Geometry: final body of the model. Coordinates: model frame, mm. A direction names the side the tool comes from. Coordinates: 2 decimals unless noted, no trailing zeros. Write each loop counter-clockwise with the first axis right and the second up, starting at its lowest first coordinate (ties: lowest second). Pieces come first, ordered by that corner, then holes. Notation, with made-up numbers: (64, -1) - (81, -1) arc R23 ccw to (81, 13) - close; hole circle Ø4 at (-30.5, 79.25). An arc over 180 degrees is marked (long way). Answer as a JSON object with one key per item and string values. Group by question number.
Item 1: Section C-C on x = -26.25. Return loops of the section in (y, z).
Item 2: Set-up query: faces 4 (the flat face through (0, 4, 2)), 5 (the cylindrical face through (-1.6, -25.9, 9.2)), 6 (the flat face through (-5, -15, 6)), 7 (the flat face through (-33, -15, 16)). Return all of +Z, -Z, +X, -X, +Y, -Y with unobstructed straight access to the full face (end or side cutting, diameter ignored); none if empty.
Item 3: Mould query, pull axis Z, two halves, no side actions, for faces 1 (the flat face through (-18, 5, 2)), 2 (the flat face through (-18, 4, 16)), 3 (the conical face through (-32.242, -21.255, 8.034)). Classes: pulls with the +Z half, pulls with the -Z half, needs draft (parallel to the pull), parting line crosses it, or undercut.
Item 4: Section B-B on z = 3. Return loops of the section in (x, y), and give its area (3 significant figures).
Item 5: Section D-D on y = -14. Return loops of the section in (x, z), and give its area (3 significant figures).
Item 6: Section A-A on y = -25. Return loops of the section in (x, z), and give its area (3 significant figures).
Item 7: First-contact query: pin 1 Ø0.6 at (y, z) = (4.5, 13) entering from +X; pin 2 Ø5 at (x, z) = (-15.5, 7) entering from -Y; pin 3 Ø4 at (y, z) = (-6, 2) entering from -X. Flat tips, straight axial feed; report the tip coordinate or a pass-through.
Item 8: Line query: line 1 along X through (y, z) = (-24, 8); line 2 along X through (y, z) = (2.45, 3); line 3 along X through (y, z) = (-25, 5.5). Output: solid intervals per line, ascending. Write a range as from..to.
Autodesk Inventor part; units mm, degrees
ref_plane "YZ Plane" through (0, 0, 0) normal (1, 0, 0) x (0, 1, 0)
ref_plane "XZ Plane" through (0, 0, 0) normal (0, 1, 0) x (-1, 0, 0)
ref_plane "XY Plane" through (0, 0, 0) normal (0, 0, 1) x (1, 0, 0)
sketch "Sketch1" plane through (0, 0, 0) normal (0, 1, 0) x (-1, 0, 0)
  line L0 (0, 0) -> (35, 0)
  line L1 (35, 0) -> (35, 6)
  line L2 (0, 6) -> (35, 6)
  line L3 (0, 0) -> (0, 6)
  line L4 (0, 6) -> (0, 0)
  line L5 (0, 3) -> (35, 3)
  line L6 (17.5, 3) -> (35, 3)
  line L7 (17.5, 3) -> (0, 3)
  point P0 (17.5, 0)
  point P1 (8.75, 3)
  point P2 (26.25, 3)
extrude "Extrusion1" add sketch "Sketch1" along normal blind 5
sketch "Sketch2" plane through (-35, 0, 6) normal (0, 0, 1) x (1, 0, 0)
  line L0 (0, 0) -> (35, 0)
  line L1 (35, 0) -> (35, 5)
  line L2 (0, 5) -> (35, 5)
  line L3 (0, 0) -> (0, 5)
extrude "Extrusion2" add sketch "Sketch2" along normal blind 10
sketch "Sketch3" plane through (0, 5, 0) normal (0, 1, 0) x (1, 0, 0)
  line L0 (0, 0) -> (0, -16)
  line L1 (0, 0) -> (-35, 0)
  line L2 (-35, 0) -> (-35, -16)
  line L3 (0, -16) -> (-35, -16)
  line L4 (-35, 0) -> (-35, -16)
  line L5 (-35, -11) -> (0, -11)
  line L6 (0, -11) -> (0, -5)
  line L7 (0, -5) -> (-35, -5)
  line L8 (-35, -5) -> (-35, -11)
  dimension "d4" = 5
  dimension "d5" = 5
extrude "Extrusion3" cut sketch "Sketch3" against normal blind 2 contours L0 L5 L2 L7
sketch "Sketch4" plane through (0, 0, 0) normal (0, -1, 0) x (1, 0, 0)
  line L0 (-35, 0) -> (0, 0)
  line L1 (0, 0) -> (0, 6)
  line L2 (-35, 6) -> (0, 6)
  line L3 (-35, 0) -> (-35, 6)
  line L4 (-35, 6) -> (-35, 0)
  line L5 (-35, 3) -> (0, 3)
  line L6 (-17.5, 3) -> (0, 3)
  line L7 (-17.5, 3) -> (-35, 3)
  point P0 (0, 0)
  point P1 (-17.5, 0)
  point P2 (-8.75, 3)
  point P3 (-26.25, 3)
hole "Hole1" at (-8.75, 0, 3) at (-26.25, 0, 3) direction (0, 1, 0) diameter 3 depth 8 tip angle 118
sketch "Sketch6" plane through (0, 0, 0) normal (0, -1, 0) x (1, 0, 0)
  circle A0 centre (-8.75, 3) radius 1.5
  circle A1 centre (-26.25, 3) radius 1.5
  line L0 (-35, 0) -> (-35, 16)
  line L1 (0, 0) -> (-35, 0)
  line L2 (0, 0) -> (0, 16)
  line L3 (-35, 16) -> (0, 16)
  line L4 (-35, 16) -> (-30, 16)
  line L5 (-30, 16) -> (-30, 0)
  line L6 (-30, 0) -> (-35, 0)
  line L7 (-35, 0) -> (-35, 16)
  line L8 (-35, 16) -> (0, 16)
  line L9 (0, 16) -> (-5, 16)
  line L10 (-5, 16) -> (-5, 0)
  line L11 (-5, 0) -> (0, 0)
  line L12 (0, 0) -> (0, 16)
  line L13 (-30, 13) -> (-5, 13)
  line L14 (-34, 14) -> (-1, 14)
  line L15 (-1, 14) -> (-1, 12)
  line L16 (-1, 12) -> (-34, 12)
  line L17 (-34, 12) -> (-34, 14)
  line L18 (-34, 14) -> (-1, 12) construction
  line L19 (-1, 14) -> (-34, 12) construction
  line L20 (-36, 17) -> (-36, 0)
  line L21 (-36, 0) -> (1, 0)
  line L22 (1, 0) -> (1, 17)
  line L23 (-36, 17) -> (1, 17)
  point P0 (-17.5, 13)
  dimension "d23" = 5
  dimension "d24" = 16
  dimension "d25" = 5
  dimension "d26" = 16
  dimension "d27" = 3
  dimension "d28" = 33
  dimension "d29" = 2
  dimension "d30" = 1
  dimension "d31" = 1
  dimension "d32" = 1
  dimension "d33" = 0
extrude "Extrusion5" add sketch "Sketch6" along normal blind 30 contours L0 L3 L5 L14 L17 L16 L1 | L10 L16 L15 L14 L3 L2 L1 | L16 L17 L14 L5 | L10 L14 L15 L16
extrude "Extrusion6" cut sketch "Sketch6" along normal blind 35 and the other way blind 1 contours L16 L17 L14 L5 | L5 L13 L10 L16 | L14 L10 L13 L5 | L10 L14 L15 L16
extrude "Extrusion7" add sketch "Sketch6" against normal up to surface (3 mm away) contours L21 L20 L23 L22 L2 L3 L0
sketch "Sketch7" plane through (0, -30, 0) normal (0, -1, 0) x (1, 0, 0)
  line L0 (-30, 12) -> (-34, 12)
  line L1 (-34, 12) -> (-34, 14)
  line L2 (-34, 14) -> (-30, 14)
  line L3 (-30, 14) -> (-30, 16)
  line L4 (-30, 16) -> (-35, 16)
  line L5 (-35, 16) -> (-35, 0)
  line L6 (-35, 0) -> (-30, 0)
  line L7 (-30, 0) -> (-30, 12)
  line L8 (-1, 12) -> (-5, 12)
  line L9 (-5, 12) -> (-5, 0)
  line L10 (-5, 0) -> (0, 0)
  line L11 (0, 0) -> (0, 16)
  line L12 (0, 16) -> (-5, 16)
  line L13 (-5, 16) -> (-5, 14)
  line L14 (-5, 14) -> (-1, 14)
  line L15 (-1, 14) -> (-1, 12)
  point P0 (0, 0)
sketch "Sketch8" plane through (0, -30, 0) normal (0, -1, 0) x (1, 0, 0)
  line L0 (-30, 12) -> (-34, 12)
  line L1 (-34, 12) -> (-34, 14)
  line L2 (-34, 14) -> (-30, 14)
  line L3 (-30, 14) -> (-30, 16)
  line L4 (-30, 16) -> (-35, 16)
  line L5 (-35, 16) -> (-35, 0)
  line L6 (-35, 0) -> (-30, 0)
  line L7 (-30, 0) -> (-30, 12)
  line L8 (-1, 12) -> (-5, 12)
  line L9 (-5, 12) -> (-5, 0)
  line L10 (-5, 0) -> (0, 0)
  line L11 (0, 0) -> (0, 16)
  line L12 (0, 16) -> (-5, 16)
  line L13 (-5, 16) -> (-5, 14)
  line L14 (-5, 14) -> (-1, 14)
  line L15 (-1, 14) -> (-1, 12)
  line L16 (-35, 16) -> (-30, 0)
  line L17 (-5, 0) -> (0, 16)
  point P0 (0, 0)
  point P1 (-32.5, 8)
  point P2 (-2.5, 8)
hole "Hole2" at (-32.5, -30, 8) at (-2.5, -30, 8) direction (0, 1, 0) diameter 3 depth 8 tip angle 118
properties part number "slide_sensor_clip" material "ABS Plastic"
Checks:
{
 "1": {"outline": "(0, 0) - (5, 0) - (5, 1.5) - (0, 1.5) - close; (0, 4.5) - (5, 4.5) - (5, 5) - (3, 5) - (3, 11) - (5, 11) - (5, 16) - (3, 16) - (3, 17) - (0, 17) - (0, 14) - (1, 14) - (1, 12) - (0, 12) - close"},
 "2": {"face 4": "+Z, -Z, +X, +Y", "face 5": "-Y", "face 6": "+Z, -Z, -Y", "face 7": "+Z, +X, -X, -Y"},
 "3": {"face 1": "needs draft", "face 2": "pulls with the +Z half", "face 3": "undercut"},
 "4": {"outline": "(-36, 0) - (-35, 0) - (-35, -30) - (-30, -30) - (-30, 0) - (-27.75, 0) - (-27.75, 5) - (-35, 5) - (-35, 3) - (-36, 3) - close; (-24.75, 0) - (-10.25, 0) - (-10.25, 5) - (-24.75, 5) - close; (-7.25, 0) - (-5, 0) - (-5, -30) - (0, -30) - (0, 0) - (1, 0) - (1, 3) - (0, 3) - (0, 5) - (-7.25, 5) - close", "area": "451 mm^2"},
 "5": {"outline": "(-35, 0) - (-30, 0) - (-30, 12) - (-34, 12) - (-34, 14) - (-30, 14) - (-30, 16) - (-35, 16) - close; (-5, 0) - (0, 0) - (0, 16) - (-5, 16) - (-5, 14) - (-1, 14) - (-1, 12) - (-5, 12) - close", "area": "144 mm^2"},
 "6": {"outline": "(-35, 0) - (-30, 0) - (-30, 12) - (-34, 12) - (-34, 14) - (-30, 14) - (-30, 16) - (-35, 16) - close; (-5, 0) - (0, 0) - (0, 16) - (-5, 16) - (-5, 14) - (-1, 14) - (-1, 12) - (-5, 12) - close; hole circle Ø3 at (-32.5, 8); hole circle Ø3 at (-2.5, 8)", "area": "130 mm^2"},
 "7": {"pin 1": "x = 0", "pin 2": "y = 0", "pin 3": "x = -35"},
 "8": {"line 1": "-35..-34, -31..-30, -5..-4, -1..0", "line 2": "-36..-27.75, -24.75..-10.25, -7.25..1", "line 3": "-35..-30, -5..0"}
}
